```python
from build123d import *

# Parameters (mm, degrees)
BOSS_EXTRUDE1_DEPTH                            = 6.35
SKETCH2_W                                      = 11.1125
SKETCH2_H                                      = 11.90625
CUT_EXTRUDE1_DEPTH                             = 7.35
SHELL1_T                                       = -1
BOSS_EXTRUDE2_REACH                            = 8.35
SKETCH5_W                                      = 5.7752
SKETCH5_H                                      = 5.7752
CBORE_FOR_2_SOCKET_HEAD_CAP_SCREW2_D           = 2.7051
CBORE_FOR_2_SOCKET_HEAD_CAP_SCREW2_CBORE_D     = 4.7625
CBORE_FOR_2_SOCKET_HEAD_CAP_SCREW2_CBORE_DEPTH = 2.1844
CUT_EXTRUDE2_DEPTH                             = 4.9276
SKETCH7_W                                      = 11.1125
SKETCH7_H                                      = 11.90625
BOSS_EXTRUDE4_DEPTH                            = 0.4224
SKETCH8_W                                      = 4.7625
SKETCH8_H                                      = 2.3876
CUT_EXTRUDE3_DEPTH                             = 2.1844
FILLET1_R                                      = 0.508


with BuildPart() as part:
    # Sketch1 → Boss-Extrude1 (new body)
    with BuildSketch(Plane.XY):
        Polygon((81.28, -96.5042297), (81.28, -72.1202297), (81.28, -70.5962297), (66.04, -70.5962297), (66.04, -72.1202297), (66.04, -96.5042297), (66.04, -98.0282297), (81.28, -98.0282297), align=None)
    extrude(amount=BOSS_EXTRUDE1_DEPTH)

    # Sketch2 → Cut-Extrude1 (cut, through all)
    with BuildSketch(Plane.XY.offset(6.35)):
        with Locations((73.66, -84.3122297)):
            Rectangle(SKETCH2_W, SKETCH2_H)
    extrude(amount=-CUT_EXTRUDE1_DEPTH, mode=Mode.SUBTRACT)

    # Shell1
    shell1_openings = [part.faces().sort_by_distance(p)[0] for p in [
        (73.66, -90.2653547, 3.175),
        (68.10375, -84.3122297, 3.175),
        (73.66, -78.3591047, 3.175),
        (79.21625, -84.3122297, 3.175),
        (73.66, -84.3122297, 0),
    ]]
    offset(amount=SHELL1_T, openings=shell1_openings, kind=Kind.INTERSECTION)

    # Sketch5 → Boss-Extrude2 (add, up to next)
    with BuildSketch(Plane(origin=(0, 0, 0), x_dir=(-1, 0, 0), z_dir=(0, 0, -1)), mode=Mode.PRIVATE) as boss_extrude2_sk1:
        with Locations((-73.66, -73.4838297)):
            Rectangle(SKETCH5_W, SKETCH5_H)
    boss_extrude2_tool1 = extrude(boss_extrude2_sk1.sketch, amount=-BOSS_EXTRUDE2_REACH, mode=Mode.PRIVATE) - part.part
    add(boss_extrude2_tool1.solids().sort_by_distance((73.66, -73.48383, 0))[0])
    # Sketch5 → Boss-Extrude2 (add, up to next)
    with BuildSketch(Plane(origin=(0, 0, 0), x_dir=(-1, 0, 0), z_dir=(0, 0, -1)), mode=Mode.PRIVATE) as boss_extrude2_sk2:
        with Locations((-73.66, -95.1406297)):
            Rectangle(SKETCH5_W, SKETCH5_H)
    boss_extrude2_tool2 = extrude(boss_extrude2_sk2.sketch, amount=-BOSS_EXTRUDE2_REACH, mode=Mode.PRIVATE) - part.part
    add(boss_extrude2_tool2.solids().sort_by_distance((73.66, -95.14063, 0))[0])

    # CBORE for #2 Socket Head Cap Screw2 (through all)
    with Locations(Plane.XY.offset(6.35)):
        with Locations((73.66, -95.6406297), (73.66, -72.9838297)):
            CounterBoreHole(CBORE_FOR_2_SOCKET_HEAD_CAP_SCREW2_D / 2, CBORE_FOR_2_SOCKET_HEAD_CAP_SCREW2_CBORE_D / 2, CBORE_FOR_2_SOCKET_HEAD_CAP_SCREW2_CBORE_DEPTH)

    # Sketch6 → Cut-Extrude2 (cut)
    with BuildSketch(Plane(origin=(0, 0, 0), x_dir=(-1, 0, 0), z_dir=(0, 0, -1))):
        with BuildLine():
            Line((-76.5476, -95.6406297), (-76.8016, -95.6406297))
            Line((-76.8016, -95.6406297), (-76.8016, -92.2530297))
            Line((-76.8016, -92.2530297), (-70.5184, -92.2530297))
            Line((-70.5184, -92.2530297), (-70.5184, -95.6406297))
            Line((-70.5184, -95.6406297), (-70.7724, -95.6406297))
            ThreePointArc((-70.7724, -95.6406297), (-73.66, -92.7530297), (-76.5476, -95.6406297))
        make_face()
        with BuildLine():
            Line((-76.8016, -72.9838297), (-76.8016, -76.3714297))
            Line((-76.8016, -76.3714297), (-70.5184, -76.3714297))
            Line((-70.5184, -76.3714297), (-70.5184, -72.9838297))
            Line((-70.5184, -72.9838297), (-70.7724, -72.9838297))
            ThreePointArc((-70.7724, -72.9838297), (-73.66, -75.8714297), (-76.5476, -72.9838297))
            Line((-76.5476, -72.9838297), (-76.8016, -72.9838297))
        make_face()
    extrude(amount=-CUT_EXTRUDE2_DEPTH, mode=Mode.SUBTRACT)

    # Sketch7 → Boss-Extrude4 (add)
    with BuildSketch(Plane(origin=(0, 0, 5.35), x_dir=(-1, 0, 0), z_dir=(0, 0, -1))):
        Polygon((-70.7724, -76.3714297), (-76.5476, -76.3714297), (-76.5476, -71.5962297), (-80.28, -71.5962297), (-80.28, -97.0282297), (-76.5476, -97.0282297), (-76.5476, -92.2530297), (-70.7724, -92.2530297), (-70.7724, -97.0282297), (-67.04, -97.0282297), (-67.04, -71.5962297), (-70.7724, -71.5962297), align=None)
        with Locations((-73.66, -84.3122297)):
            Rectangle(SKETCH7_W, SKETCH7_H, mode=Mode.SUBTRACT)
    extrude(amount=BOSS_EXTRUDE4_DEPTH)

    # Sketch8 → Cut-Extrude3 (cut)
    with BuildSketch(Plane.XY.offset(6.35)):
        with Locations((73.66, -96.8344297)):
            Rectangle(SKETCH8_W, SKETCH8_H)
        with Locations((73.66, -71.7900297)):
            Rectangle(SKETCH8_W, SKETCH8_H)
    extrude(amount=-CUT_EXTRUDE3_DEPTH, mode=Mode.SUBTRACT)

    # Fillet1
    fillet1_edges = [part.edges().sort_by_distance(p)[0] for p in [
        (73.66, -93.2593797, 6.35),
        (78.660625, -70.5962297, 6.35),
        (81.28, -98.0282297, 3.175),
        (66.04, -98.0282297, 3.175),
        (66.04, -70.5962297, 3.175),
        (81.28, -70.5962297, 3.175),
        (66.04, -84.3122297, 6.35),
        (78.660625, -98.0282297, 6.35),
        (76.04125, -96.8344297, 6.35),
        (71.27875, -96.8344297, 6.35),
        (73.66, -75.3650797, 6.35),
        (68.659375, -70.5962297, 6.35),
        (71.27875, -71.7900297, 6.35),
        (76.04125, -71.7900297, 6.35),
        (68.659375, -98.0282297, 6.35),
        (79.21625, -90.2653547, 5.6388),
        (68.10375, -90.2653547, 5.6388),
        (68.10375, -78.3591047, 5.6388),
        (79.21625, -78.3591047, 5.6388),
        (73.66, -90.2653547, 6.35),
        (79.21625, -84.3122297, 6.35),
        (73.66, -78.3591047, 6.35),
        (68.10375, -84.3122297, 6.35),
        (81.28, -84.3122297, 6.35),
    ]]
    fillet(fillet1_edges, radius=FILLET1_R)


solid = part.part
```
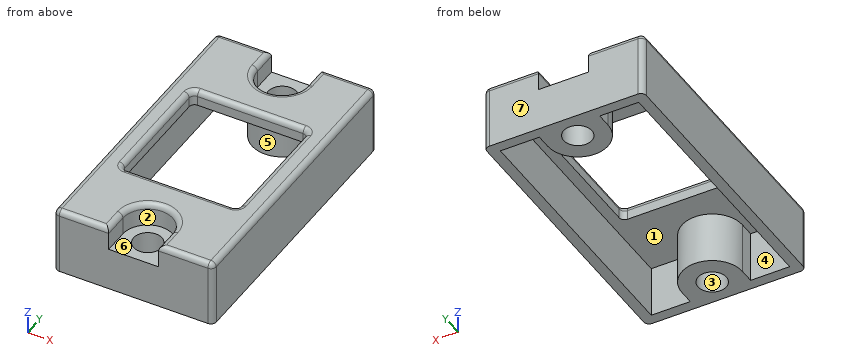
Here's how the part is built. I have some questions about the finished solid (model axes, mm). Face numbers are marked on the shaded views. A direction names the side the tool comes from. Coordinates: 2 decimals unless noted, no trailing zeros. Write each loop counter-clockwise with the first axis right and the second up, starting at its lowest first coordinate (ties: lowest second). Pieces come first, ordered by that corner, then holes. Notation, with made-up numbers: M -26.75,-26.75 L 6.25,-26.75 A18 cw 6.25,-22.75 Z; hole C 51.25,64 d3. An arc over 180 degrees is marked long. Answer as CSV lines item,"result". Start each with the question number.
Q1. Will these pins go through, and if not, where does the flat tip stop? pin 1 Ø2 at (x, y) = (73.66, -72.98) entering from -Z; pin 2 Ø0.7 at (x, z) = (74.5, 5) entering from -Y.
Q2. For the marked faces 1, 2 and 3, which set-ups out of +Z, -Z, +X, -X, +Y, -Y let a thin tool reach every point of the face, with its end or its side?
Q3. Suppose I cut it at D-D, the plane z = 0.75. List the corners of the cut face in (x, y) for me.
Q4. Suppose I cut it at B-B, the plane y = -79.25. List the corners of the cut face in (x, z) for me, then the cut area to 3 significant figures.
Q5. If we mould it in two halves opening along Y, with no side actions, what happens to the marked faces 4, 5, 6 and 7? For each: pulls with the +Y half, pulls with the -Y half, needs draft (parallel to the pull), parting line crosses it, or undercut.
Q6. I need wall thicknesses on probe 1 along X at (y, z) = (-73, 1.5); probe 2 along Y at (x, z) = (73.66, 2.5); probe 3 along Y at (x, z) = (68.25, 1.25). Which ranges of each line are inside material? Lowest first, please. Write a range as [from, to].
Q7. Suppose I cut it at C-C, the plane z = 5.5. List the corners of the cut face in (x, y) for me, then the cut area to 3 significant figures.
Q8. Suppose I cut it at A-A, the plane x = 73.66. List the corners of the cut face in (y, z) for me.
Entries:
1,pin 1,"passes through"
1,pin 2,"stops at y = -93.58"
2,face 1,"-Z"
2,face 2,"+Z, -Y"
2,face 3,"+Z, -Z"
3,outline,"M 66.04,-97.52 A0.51 ccw 66.55,-98.03 L 80.77,-98.03 A0.51 ccw 81.28,-97.52 L 81.28,-71.1 A0.51 ccw 80.77,-70.6 L 66.55,-70.6 A0.51 ccw 66.04,-71.1 Z; hole M 67.04,-97.03 L 70.77,-97.03 L 70.77,-95.64 A2.89 cw 76.55,-95.64 L 76.55,-97.03 L 80.28,-97.03 L 80.28,-71.6 L 76.55,-71.6 L 76.55,-72.98 A2.89 cw 70.77,-72.98 L 70.77,-71.6 L 67.04,-71.6 Z; hole C 73.66,-95.64 d2.71; hole C 73.66,-72.98 d2.71"
4,outline,"M 66.04,0 L 67.04,0 L 67.04,4.93 L 68.1,4.93 L 68.1,5.84 A0.51 ccw 67.6,6.35 L 66.55,6.35 A0.51 ccw 66.04,5.84 Z; M 79.22,4.93 L 80.28,4.93 L 80.28,0 L 81.28,0 L 81.28,5.84 A0.51 ccw 80.77,6.35 L 79.72,6.35 A0.51 ccw 79.22,5.84 Z"
4,area,"15.5 mm²"
5,face 4,"undercut"
5,face 5,"undercut"
5,face 6,"needs draft"
5,face 7,"pulls with the +Y half"
6,probe 1,"x = [66.04, 67.04], [70.77, 72.31], [75.01, 76.55], [80.28, 81.28]"
6,probe 2,"y = [-98.03, -96.99], [-94.29, -92.75], [-75.87, -74.34], [-71.63, -70.6]"
6,probe 3,"y = [-98.03, -97.03], [-71.6, -70.6]"
7,outline,"M 66.04,-97.52 A0.51 ccw 66.55,-98.03 L 71.28,-98.03 L 71.28,-95.64 A2.38 cw 76.04,-95.64 L 76.04,-98.03 L 80.77,-98.03 A0.51 ccw 81.28,-97.52 L 81.28,-71.1 A0.51 ccw 80.77,-70.6 L 76.04,-70.6 L 76.04,-72.98 A2.38 cw 71.28,-72.98 L 71.28,-70.6 L 66.55,-70.6 A0.51 ccw 66.04,-71.1 Z; hole M 68.1,-89.76 A0.51 ccw 68.61,-90.27 L 78.71,-90.27 A0.51 ccw 79.22,-89.76 L 79.22,-78.87 A0.51 ccw 78.71,-78.36 L 68.61,-78.36 A0.51 ccw 68.1,-78.87 Z"
7,area,"245 mm²"
8,outline,"M -98.03,0 L -96.99,0 L -96.99,4.17 L -98.03,4.17 Z; M -94.29,0 L -92.75,0 L -92.75,4.93 L -90.27,4.93 L -90.27,5.84 A0.51 ccw -90.77,6.35 L -92.75,6.35 A0.51 ccw -93.26,5.84 L -93.26,4.17 L -94.29,4.17 Z; M -78.36,4.93 L -75.87,4.93 L -75.87,0 L -74.34,0 L -74.34,4.17 L -75.37,4.17 L -75.37,5.84 A0.51 ccw -75.87,6.35 L -77.85,6.35 A0.51 ccw -78.36,5.84 Z; M -71.63,0 L -70.6,0 L -70.6,4.17 L -71.63,4.17 Z"
